from build123d import *

# Parameters (mm, degrees)
SKETCH_1_W          = 65.34
SKETCH_1_H          = 52.4
EXTRUDE_2_DEPTH     = 5.1
SKETCH_1_5_W        = 64.34
SKETCH_1_5_H        = 51.4
CUT_EXTRUDE_2_DEPTH = 4.6
SKETCH_2_W          = 20.4
SKETCH_2_H          = 1.1
SKETCH_2_W_2        = 20.39
SKETCH_2_W_3        = 17.75
CUT_EXTRUDE_3_DEPTH = 56.4
SKETCH_9_W          = 23.6
SKETCH_9_H          = 1.1
CUT_EXTRUDE_4_DEPTH = 4.9
CUT_EXTRUDE_6_DEPTH = 4.9


with BuildPart() as part:
    # 草图1 → 凸台-拉伸2 (new body)
    with BuildSketch(Plane(origin=(0, 0, 0), x_dir=(1, 0, 0), z_dir=(0, 1, 0))):
        with Locations((32.67, 26.2)):
            Rectangle(SKETCH_1_W, SKETCH_1_H)
    extrude(amount=EXTRUDE_2_DEPTH)

    # 草图1<5> → 切除-拉伸2 (cut)
    with BuildSketch(Plane(origin=(0, 0, 0), x_dir=(1, 0, 0), z_dir=(0, 1, 0))):
        with Locations((32.67, 26.2)):
            Rectangle(SKETCH_1_5_W, SKETCH_1_5_H)
    extrude(amount=CUT_EXTRUDE_2_DEPTH, mode=Mode.SUBTRACT)

    # 草图2 → 切除-拉伸3 (cut)
    with BuildSketch(Plane.XY):
        with Locations((12, 0.55)):
            Rectangle(SKETCH_2_W, SKETCH_2_H)
        with Locations((33.995, 0.55)):
            Rectangle(SKETCH_2_W_2, SKETCH_2_H)
        with Locations((54.665, 0.55)):
            Rectangle(SKETCH_2_W_3, SKETCH_2_H)
    extrude(amount=-CUT_EXTRUDE_3_DEPTH, mode=Mode.SUBTRACT)

    # 草图9 → 切除-拉伸4 (cut)
    with BuildSketch(Plane(origin=(65.34, 0, 0), x_dir=(0, 0, -1), z_dir=(1, 0, 0))):
        with Locations((13.6, 0.55)):
            Rectangle(SKETCH_9_W, SKETCH_9_H)
        Polygon((27, 0), (50.6, 0), (50.6, 1.1), (45, 1.1), (45, 4.1), (40, 4.1), (40, 1.1), (27, 1.1), align=None)
    extrude(amount=-CUT_EXTRUDE_4_DEPTH, mode=Mode.SUBTRACT)

    # 草图13 → 切除-拉伸6 (cut)
    with BuildSketch(Plane.ZY):
        Polygon((-50.6, 0), (-50.6, 1.1), (-41.77, 1.1), (-41.77, 4.1), (-18.8, 4.1), (-18.8, 1.1), (-1.8, 1.1), (-1.8, 0), align=None)
    extrude(amount=-CUT_EXTRUDE_6_DEPTH, mode=Mode.SUBTRACT)


solid = part.part
The model under review builds one solid part; all positions refer to its coordinate system, in mm. A direction names the side the tool comes from. Round coordinates to 2 decimals unless told otherwise and drop trailing zeros. Loops run counter-clockwise (first coordinate to the right, second up) from the corner with the lowest first, then second, coordinate; pieces in that order, holes last. Notation, with made-up numbers: M 33.5,35 L 47.5,35 A31 ccw 47.5,61 Z; hole C 10,3.25 d7. An arc over 180 degrees is marked long. Answer as CSV lines item,"result". Start each with the question number.
Item 1: Mouldability with a two-part tool opening along X and no side actions: class faces 1 (the face through (0, 4.8, -25.8)), 2 (the face through (0.3, 0, -51.7)), 3 (the face through (0.5, 4.3, -25.8)), 4 (the face through (65.34, 3, -26)) as released by +X, released by -X, zero draft, split by the parting line, or undercut.
Item 2: Consider section B-B (z = -35.5). Write out the cut boundary in (x, y).
Item 3: Insertion check: P1, Ø8, axis at x = 11.5, z = -20, coming from the -Y side; P2, Ø0.6, axis at x = 0.5, z = -6, coming from the -Y side. Each pin has a flat end and moves straight along its axis. Give the tip position at first contact, or say it passes through.
Item 4: Consider section A-A (y = 1.95). Write out the cut boundary in (x, z).
Item 5: For faces 5 (the face through (0.3, 0, -0.7)), 6 (the face through (32, 4.6, -27)), list the 3-axis set-ups (+Z, -Z, +X, -X, +Y, -Y) from which the entire face can be reached by the end or side of a thin tool; tool diameter is ignored.
Item 6: Wall thickness on line 1 (Z direction, x = 11, y = 3.05); line 2 (X direction, y = 2.45, z = -13.5); line 3 (Y direction, x = 4, z = -26.5): over which ranges is each line inside the solid? List them lowest first. Write a range as [from, to].
Item 7: Consider section C-C (x = 58.5). Write out the cut boundary in (y, z).
Answer:
1,face 1,"released by -X"
1,face 2,"zero draft"
1,face 3,"undercut"
1,face 4,"released by +X"
2,outline,"M 0,4.1 L 0.5,4.1 L 0.5,4.6 L 64.84,4.6 L 64.84,1.1 L 65.34,1.1 L 65.34,5.1 L 0,5.1 Z"
3,P1,"stops at y = 4.6"
3,P2,"stops at y = 1.1"
4,outline,"M 0,-52.4 L 65.34,-52.4 L 65.34,-45 L 64.84,-45 L 64.84,-51.9 L 0.5,-51.9 L 0.5,-41.77 L 0,-41.77 Z; M 0,-18.8 L 0.5,-18.8 L 0.5,-0.5 L 64.84,-0.5 L 64.84,-40 L 65.34,-40 L 65.34,0 L 0,0 Z"
5,face 5,"+Z, -Z, +X, -X, -Y"
5,face 6,"-Y"
6,line 1,"z = [-52.4, -51.9], [-0.5, 0]"
6,line 2,"x = [0, 0.5], [64.84, 65.34]"
6,line 3,"y = [4.6, 5.1]"
7,outline,"M 1.1,-52.4 L 5.1,-52.4 L 5.1,0 L 1.1,0 L 1.1,-0.5 L 4.6,-0.5 L 4.6,-51.9 L 1.1,-51.9 Z"
